Input: part model. Units: mm. Frame: model coordinates. A direction names the side the tool comes from. Give positions to 0.01 mm unless a question says otherwise; leave off trailing zeros. Write each loop counter-clockwise with the first axis right and the second up, starting at its lowest first coordinate (ties: lowest second). Pieces come first, ordered by that corner, then holes. Notation, with made-up numbers: (40.5, 40.25) - (83.5, 40.25) arc R17 ccw to (83.5, 52.25) - close; hole circle Ø7 at (63, -33.5). An arc over 180 degrees is marked (long way). Answer as CSV lines item,"result". Start each with the question number.
from build123d import *

# Parameters (mm, degrees)
BASIS_BLECH1_DEPTH              = 173
BLECHKANTENRAND1_START          = -173
BLECHKANTENRAND1_DEPTH          = 346
BLECHKANTENRAND1_2_DEPTH        = 346
VERRUNDUNG1_R                   = 2
SKIZZE19_W                      = 20
SKIZZE19_H                      = 1
AUFSATZ_LINEAR_AUSTRAGEN1_DEPTH = 16
VERRUNDUNG2_R                   = 2


# Read off the part's stored shape, not the designer's step: Blechkantenrand1
# Sheet-metal steps are written as plain solids
with BuildPart() as part:
    # Skizze1 → Basis-Blech1 (new, symmetric)
    with BuildSketch(Plane(origin=(0, 0, 0), x_dir=(0, 0, -1), z_dir=(1, 0, 0))):
        with BuildLine():
            Line((0, 0), (0, 34.544365081))
            ThreePointArc((0, 34.544365081), (0.083732514, 34.965316857), (0.322182541, 35.322182541))
            Line((0.322182541, 35.322182541), (10.040916293, 45.040916293))
            Line((10.040916293, 45.040916293), (10.748023074, 44.333809512))
            Line((10.748023074, 44.333809512), (1.029289322, 34.61507576))
            ThreePointArc((1.029289322, 34.61507576), (1.007612047, 34.582633425), (1, 34.544365081))
            Line((1, 34.544365081), (1, 0))
            Line((1, 0), (0, 0))
        make_face()
    extrude(amount=BASIS_BLECH1_DEPTH, both=True)

    # Blechkantenrand1 outline → Blechkantenrand1 (cut)
    with BuildSketch(Plane.YZ.offset(BLECHKANTENRAND1_START)):
        with BuildLine():
            Line((45.040916293, -10.040916293), (45.040074021, -10.040074021))
            ThreePointArc((45.040074021, -10.040074021), (44.308802418, -10.312801004), (43.591347391, -10.005560954))
            Line((43.591347391, -10.005560954), (44.333809512, -10.748023074))
            Line((44.333809512, -10.748023074), (45.040916293, -10.040916293))
        make_face()
    extrude(amount=BLECHKANTENRAND1_DEPTH, mode=Mode.SUBTRACT)

    # Blechkantenrand1 2 outline → Blechkantenrand1 2 (add)
    with BuildSketch(Plane.YZ.offset(BLECHKANTENRAND1_START)):
        with BuildLine():
            Line((40.161879503, -3.606244584), (39.454772721, -4.313351365))
            Line((39.454772721, -4.313351365), (44.369164851, -9.227743494))
            ThreePointArc((44.369164851, -9.227743494), (44.369164852, -9.298454172), (44.298454173, -9.298454173))
            Line((44.298454173, -9.298454173), (45.040074021, -10.040074021))
            ThreePointArc((45.040074021, -10.040074021), (45.383511682, -9.288105927), (45.076271632, -8.520636713))
            Line((45.076271632, -8.520636713), (40.161879503, -3.606244584))
        make_face()
    extrude(amount=BLECHKANTENRAND1_2_DEPTH)

    # Verrundung1
    verrundung1_edges = [part.edges().sort_by_distance(p)[0] for p in [
        (173, 0, -0.5),
        (-173, 39.808326112, -3.959797974),
        (173, 39.808326112, -3.959797974),
        (-173, 0, -0.5),
    ]]
    fillet(verrundung1_edges, radius=VERRUNDUNG1_R)

    # Skizze19 → Aufsatz-Linear austragen1 (add)
    with BuildSketch(Plane.XZ):
        with Locations((-63, -0.5)):
            Rectangle(SKIZZE19_W, SKIZZE19_H)
        with Locations((77, -0.5)):
            Rectangle(SKIZZE19_W, SKIZZE19_H)
    extrude(amount=AUFSATZ_LINEAR_AUSTRAGEN1_DEPTH)

    # Verrundung2
    verrundung2_edges = [part.edges().sort_by_distance(p)[0] for p in [
        (-73, 0, -0.5),
        (-53, 0, -0.5),
        (-73, -16, -0.5),
        (-53, -16, -0.5),
        (67, 0, -0.5),
        (87, 0, -0.5),
        (67, -16, -0.5),
        (87, -16, -0.5),
    ]]
    fillet(verrundung2_edges, radius=VERRUNDUNG2_R)


solid = part.part
1) Cut plane C-C on x = -24. Output: boundary loops of the cut face in (y, z).
2) Cut plane A-A on y = -9.5. Output: boundary loops of the cut face in (x, z).
3) Pull-direction query (Y, two-part tool) for faces 1 (the flat face through (-173, 25.2, -0.5)), 2 (the flat face through (2, 39, -4)), 3 (the flat face through (2.422, 39.166, -5.58)); classes: +Y half, -Y half, draft (parallel to the pull), parting line (faces both ways), or undercut.
4) Cut plane D-D on y = 12.5. Output: boundary loops of the cut face in (x, z), and give its area (3 significant figures).
5) Cut plane B-B on x = 73. Output: boundary loops of the cut face in (y, z).
6) Material intervals for line 1 (Z direction, x = -62, y = -8); line 2 (Y direction, x = -120, z = -10); line 3 (Y direction, x = 3.5, z = -2), sorted ascending. Write a range as from..to.
7) Contact query for flat-ended pins moving along their axis: P1, Ø1.1, axis at y = -6.5, z = -0.5, coming from the -X side; P2, Ø0.8, axis at x = 14, z = -0.5, coming from the -Y side; P3, Ø4, axis at x = -37, y = 30.5, coming from the -Z side. Output: stop coordinate, or through.
8) Reachability of faces 4 (the flat face through (173, 25.2, -0.5)), 5 (the flat face through (2, 15, -1)) from +Z, -Z, +X, -X, +Y, -Y: full face, straight path, thin tool, end or side. Return the list, or none.
Numbers:
1,outline,"(0, -1) - (34.54, -1) arc R0.1 cw to (34.62, -1.03) - (43.59, -10.01) arc R1.05 ccw to (45.08, -8.52) - (40.16, -3.61) - (39.45, -4.31) - (44.37, -9.23) arc R0.05 cw to (44.3, -9.3) - (35.32, -0.32) arc R1.1 ccw to (34.54, 0) - (0, 0) - close"
2,outline,"(-73, -1) - (-53, -1) - (-53, 0) - (-73, 0) - close; (67, -1) - (87, -1) - (87, 0) - (67, 0) - close"
3,face 1,"draft"
3,face 2,"undercut"
3,face 3,"-Y half"
4,outline,"(-173, -1) - (173, -1) - (173, 0) - (-173, 0) - close"
4,area,"346 mm²"
5,outline,"(-16, -1) - (34.54, -1) arc R0.1 cw to (34.62, -1.03) - (43.59, -10.01) arc R1.05 ccw to (45.08, -8.52) - (40.16, -3.61) - (39.45, -4.31) - (44.37, -9.23) arc R0.05 cw to (44.3, -9.3) - (35.32, -0.32) arc R1.1 ccw to (34.54, 0) - (-16, 0) - close"
6,line 1,"z = -1..0"
6,line 2,"y = 43.59..45.08"
6,line 3,"y = 35.59..37"
7,P1,"stops at x = -73"
7,P2,"stops at y = 0"
7,P3,"stops at z = -1"
8,face 4,"+Z, -Z, +X, +Y, -Y"
8,face 5,"-Z, +X, -X, -Y"
